Source: CAD feature listing. Evaluate the final solid. Frame: model axes, mm. Face numbers are marked on the shaded views. A direction names the side the tool comes from. Give positions to 0.01 mm unless a question says otherwise; leave off trailing zeros. Order: outer loops, then holes, each group sorted by start corner. A loop starts at its lowest first (then second) coordinate and runs counter-clockwise, first axis right, second up. Notation, with made-up numbers: M 51,-4.75 L 80,-4.75 A11 cw 80,3.25 Z; hole C 47,57.5 d7. An arc over 180 degrees is marked long. Return JSON: item names as keys, results as strings.
from build123d import *

# Parameters (mm, degrees)
F1_DEPTH  = 25.4
F3_DEPTH  = 12.7
F4_R      = 25.4
F5_DEPTH  = 76.2
F6_R      = 12.7
F7_DEPTH  = 76.201
F8_W      = 25.4
F8_H      = 12.7
F9_DEPTH  = 76.201
F11_DEPTH = 50.801


with BuildPart() as f1:
    # F0 (on Front) → F1 (new body)
    with BuildSketch(Plane.XZ):
        Polygon((0, 50.8), (0, 0), (38.1, 0), align=None)
    extrude(amount=-F1_DEPTH)

    # F2 (on face) → F3 (join)
    with BuildSketch(Plane.XZ):
        Polygon((38.1, 0), (0, 50.8), (0, 0), align=None)
    extrude(amount=F3_DEPTH)

    # F4 (on face) → F5 (join)
    with BuildSketch(Plane(origin=(0, 0, 0), x_dir=(0, -1, 0), z_dir=(-1, 0, 0))):
        Circle(F4_R)
    extrude(amount=-F5_DEPTH)

    # F6 (on face) → F7 (cut, through all)
    with BuildSketch(Plane(origin=(0, 0, 0), x_dir=(0, -1, 0), z_dir=(-1, 0, 0))):
        Circle(F6_R)
    extrude(amount=-F7_DEPTH, mode=Mode.SUBTRACT)

    # F8 (on face) → F9 (cut, through all)
    with BuildSketch(Plane(origin=(0, 0, 0), x_dir=(0, -1, 0), z_dir=(-1, 0, 0))):
        with Locations((0, 44.45)):
            Rectangle(F8_W, F8_H)
    extrude(amount=-F9_DEPTH, mode=Mode.SUBTRACT)

    # F10 (on face) → F11 (cut, through all)
    with BuildSketch(Plane(origin=(0, 25.4, 0), x_dir=(-1, 0, 0), z_dir=(0, 1, 0))):
        Polygon((-50.951158, 25.4), (-76.351158, 25.4), (-76.351158, 9.525), (-63.651158, 9.525), (-63.651158, -9.525), (-50.951158, -9.525), align=None)
    extrude(amount=-F11_DEPTH, mode=Mode.SUBTRACT)


solid = f1.part
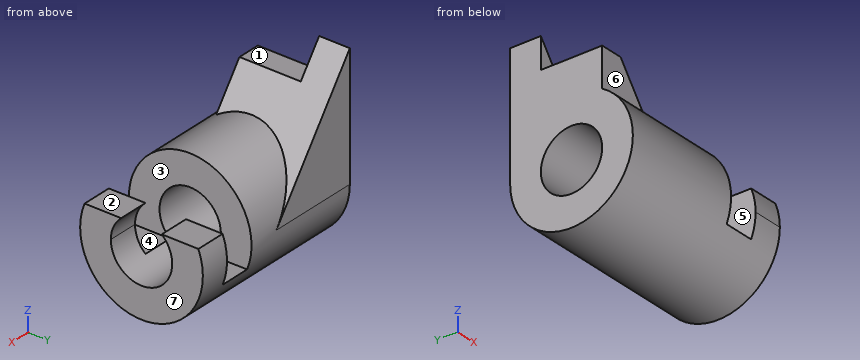
1. Section query D-D (x = 65). Return loops of the section in (y, z) (3 decimals).
Evaluation:
{"outline": "M -23.546,9.525 A25.4 ccw long 23.546,9.525 L 8.4,9.525 A12.7 cw long -8.4,9.525 Z"}
2. Set-up query: the marked faces 1, 2 and 3. Return all of +Z, -Z, +X, -X, +Y, -Y with unobstructed straight access to the full face (end or side cutting, diameter ignored); none if empty.
Evaluation:
{"face 1": "+Z, +X, -X, -Y", "face 2": "+Z, +X, +Y, -Y", "face 3": "+Z, +Y, -Y"}
3. Ray query, probe 1 along Z at (x, y) = (46.5, 0); probe 2 along X at (y, z) = (0, 22). Return the intervals inside material, ascending.
Evaluation:
{"probe 1": "z = -25.4 to -12.7, 12.7 to 25.4", "probe 2": "x = 0 to 50.95"}
4. First-contact query: pin 1 (6 mm diameter, centred on x = 14, y = 5.5, fed in from -Z); pin 2 (5 mm diameter, centred on x = 58.5, y = 2.5, fed in from +Z); pin 3 (10 mm diameter, centred on x = 59, y = 13.5, fed in from +Z) (3 decimals); pin 4 (10.5 mm diameter, centred on y = 4, z = 3.5, fed in from +X). Flat tips, straight axial feed; report the tip coordinate or a pass-through.
Evaluation:
{"pin 1": "stops at z = -25.28", "pin 2": "stops at z = -11.67", "pin 3": "stops at z = 9.525", "pin 4": "passes through"}
5. Section query A-A (y = 0). Return loops of the section in (x, z) (3 decimals), then the cut area to 3 significant figures.
Evaluation:
{"outline": "M 0,-25.4 L 76.2,-25.4 L 76.2,-12.7 L 0,-12.7 Z; M 0,12.7 L 50.951,12.7 L 50.951,25.4 L 19.05,25.4 L 9.525,38.1 L 0,38.1 Z", "area": "1,800 mm^2"}
6. Section query C-C (x = 13). Return loops of the section in (y, z), then the cut area to 3 significant figures.
Evaluation:
{"outline": "M -12.7,22 A25.4 ccw long 25.4,0 L 25.4,33.47 L -12.7,33.47 Z; hole C 0,0 d25.4", "area": "1,980 mm^2"}
7. Section query B-B (y = 10). Return loops of the section in (x, z) (1 decimal).
Evaluation:
{"outline": "M 0,-23.3 L 76.2,-23.3 L 76.2,-7.8 L 63.7,-7.8 L 63.7,-9.5 L 51,-9.5 L 51,-7.8 L 0,-7.8 Z; M 0,7.8 L 51,7.8 L 51,23.3 L 20.6,23.3 L 9.5,38.1 L 0,38.1 Z; M 63.7,7.8 L 76.2,7.8 L 76.2,9.5 L 63.7,9.5 Z"}
8. Draft query along X for the marked faces 4, 5, 6 and 7. Return one class per face: pulls with the +X half, pulls with the -X half, needs draft (parallel to the pull), parting line crosses it, or undercut.
Evaluation:
{"face 4": "undercut", "face 5": "undercut", "face 6": "needs draft", "face 7": "pulls with the +X half"}
